Geometry check sheet. Reference: drawing and pictorial views, mm from the part's lowest x, y, z. Round coordinates to 2 decimals unless told otherwise and drop trailing zeros. Answer in a Markdown table with one row per item. Add a question column.
1. Go/stop test with flat-tipped pins: pin 1 Ø5 at (x, z) = (30, 2.5) entering from -Y; pin 2 Ø4 at (x, z) = (10.5, 9.5) entering from +Y; pin 3 Ø1 at (y, z) = (5, 2.5) entering from +X (1 decimal). Record where each tip stops, or that it passes through.
2. Draft check along Y on the marked faces 1, 2 and 3. Enter one of: pulls with the +Y half, pulls with the -Y half, needs draft (parallel to the pull), parting line crosses it, or undercut.
3. Material ranges on probe 1 along Y at (x, z) = (17, 6.25); probe 2 along X at (y, z) = (15.5, 8) (1 decimal); probe 3 along Y at (x, z) = (24.5, 8) (1 decimal), recorded low to high.
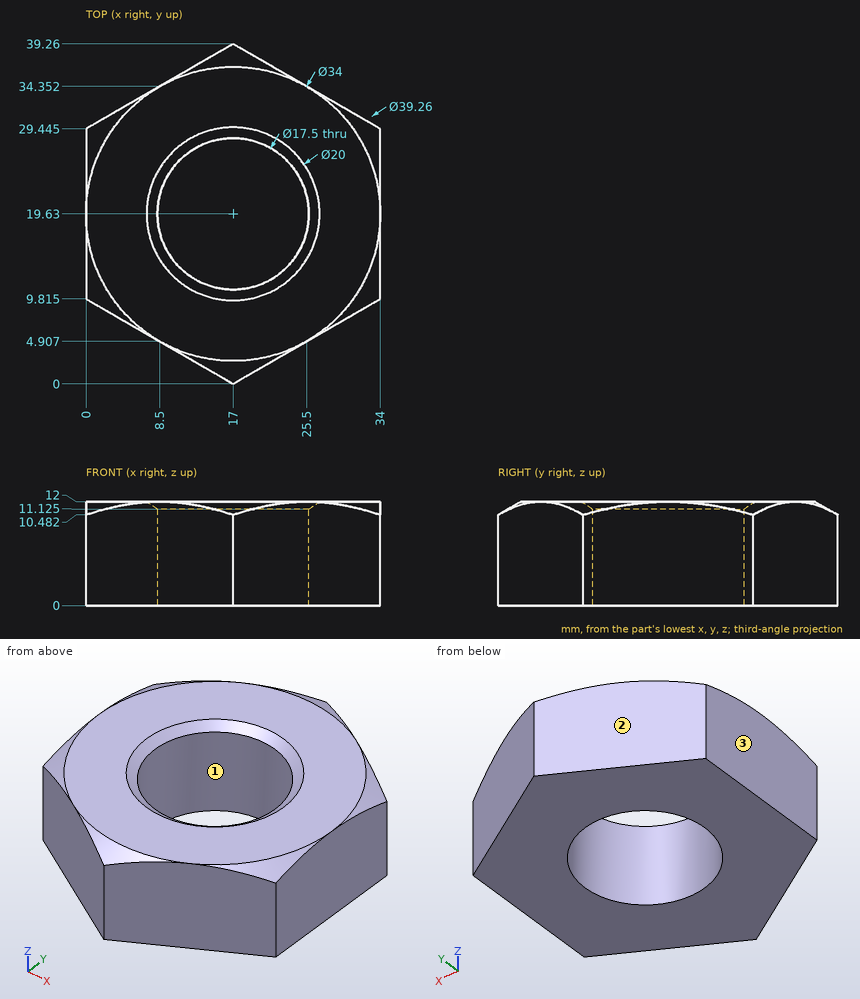
Geometry check:
| question | item | result |
|---|---|---|
| 1 | pin 1 | stops at y = 6.06 |
| 1 | pin 2 | stops at y = 36.66 |
| 1 | pin 3 | stops at x = 26.5 |
| 2 | face 1 | undercut |
| 2 | face 2 | pulls with the +Y half |
| 2 | face 3 | needs draft |
| 3 | probe 1 | y = 0 to 10.88, 28.38 to 39.26 |
| 3 | probe 2 | x = 0 to 9.3, 24.7 to 34 |
| 3 | probe 3 | y = 4.3 to 15.1, 24.1 to 34.9 |
